from build123d import *

# Parameters (mm, degrees)
SM_BASE_FLANGE_1_DEPTH    = 185
CUT_EXTRUDE_1_REACH       = 197.768
SKETCH_6_R                = 5
SM_EDGE_FLANGE_1_DEPTH    = 49.2634
HOLE_WIZARD_M3_2_D        = 3
CUT_EXTRUDE_START         = -2.7366
CUT_EXTRUDE_6_OUTLINE_W   = 21
CUT_EXTRUDE_6_OUTLINE_H   = 20
CUT_EXTRUDE_6_OUTLINE_H_2 = 19.2634
CUT_EXTRUDE_6_DEPTH       = 2.7366
HOLE_WIZARD_3_5_3_5_1_D   = 3.5
HOLE_WIZARD_7_0_7_1_D     = 7
HOLE_WIZARD_7_0_7_1_DEPTH = 6
HOLE_WIZARD_7_0_7_1_TIP   = 2.103012167
M3X0_5_1_D                = 2.5


# Read off the part's stored shape, not the designer's step: 除料-伸長6
# Sheet-metal steps are written as plain solids
with BuildPart() as part:
    # Sketch 1 → 基材-凸緣1 (new body)
    with BuildSketch(Plane.XY):
        with BuildLine():
            Line((0, -50), (0, -0.7366))
            ThreePointArc((0, -0.7366), (-0.215745145, -0.215745145), (-0.7366, 0))
            Line((-0.7366, 0), (-40, 0))
            Line((-40, 0), (-40, 2))
            Line((-40, 2), (-0.7366, 2))
            ThreePointArc((-0.7366, 2), (1.198468417, 1.198468417), (2, -0.7366))
            Line((2, -0.7366), (2, -50))
            Line((2, -50), (0, -50))
        make_face()
    extrude(amount=SM_BASE_FLANGE_1_DEPTH)

    # 草圖6 → 除料-伸長1 (cut, up to next)
    with BuildSketch(Plane.ZY, mode=Mode.PRIVATE) as cut_extrude_1_sk1:
        with Locations(Location((170, -25, 0), (0, 0, 270))):
            Circle(SKETCH_6_R)
    cut_extrude_1_tool1 = extrude(cut_extrude_1_sk1.sketch, amount=-CUT_EXTRUDE_1_REACH, mode=Mode.PRIVATE) & part.part
    # 草圖6 → 除料-伸長1 (cut, up to next)
    with BuildSketch(Plane.ZY, mode=Mode.PRIVATE) as cut_extrude_1_sk2:
        with BuildLine():
            Line((37, -12), (43, -12))
            ThreePointArc((43, -12), (56, -25), (43, -38))
            Line((43, -38), (37, -38))
            ThreePointArc((37, -38), (24, -25), (37, -12))
        make_face()
    cut_extrude_1_tool2 = extrude(cut_extrude_1_sk2.sketch, amount=-CUT_EXTRUDE_1_REACH, mode=Mode.PRIVATE) & part.part
    # 草圖6 → 除料-伸長1 (cut, up to next)
    with BuildSketch(Plane.ZY, mode=Mode.PRIVATE) as cut_extrude_1_sk3:
        with BuildLine():
            Line((58, -8.25), (64, -8.25))
            ThreePointArc((64, -8.25), (65.75, -10), (64, -11.75))
            Line((64, -11.75), (58, -11.75))
            ThreePointArc((58, -11.75), (56.25, -10), (58, -8.25))
        make_face()
    cut_extrude_1_tool3 = extrude(cut_extrude_1_sk3.sketch, amount=-CUT_EXTRUDE_1_REACH, mode=Mode.PRIVATE) & part.part
    # 草圖6 → 除料-伸長1 (cut, up to next)
    with BuildSketch(Plane.ZY, mode=Mode.PRIVATE) as cut_extrude_1_sk4:
        with BuildLine():
            Line((16, -8.25), (22, -8.25))
            ThreePointArc((22, -8.25), (23.75, -10), (22, -11.75))
            Line((22, -11.75), (16, -11.75))
            ThreePointArc((16, -11.75), (14.25, -10), (16, -8.25))
        make_face()
    cut_extrude_1_tool4 = extrude(cut_extrude_1_sk4.sketch, amount=-CUT_EXTRUDE_1_REACH, mode=Mode.PRIVATE) & part.part
    # 草圖6 → 除料-伸長1 (cut, up to next)
    with BuildSketch(Plane.ZY, mode=Mode.PRIVATE) as cut_extrude_1_sk5:
        with BuildLine():
            Line((16, -38.25), (22, -38.25))
            ThreePointArc((22, -38.25), (23.75, -40), (22, -41.75))
            Line((22, -41.75), (16, -41.75))
            ThreePointArc((16, -41.75), (14.25, -40), (16, -38.25))
        make_face()
    cut_extrude_1_tool5 = extrude(cut_extrude_1_sk5.sketch, amount=-CUT_EXTRUDE_1_REACH, mode=Mode.PRIVATE) & part.part
    # 草圖6 → 除料-伸長1 (cut, up to next)
    with BuildSketch(Plane.ZY, mode=Mode.PRIVATE) as cut_extrude_1_sk6:
        with BuildLine():
            Line((58, -38.25), (64, -38.25))
            ThreePointArc((64, -38.25), (65.75, -40), (64, -41.75))
            Line((64, -41.75), (58, -41.75))
            ThreePointArc((58, -41.75), (56.25, -40), (58, -38.25))
        make_face()
    cut_extrude_1_tool6 = extrude(cut_extrude_1_sk6.sketch, amount=-CUT_EXTRUDE_1_REACH, mode=Mode.PRIVATE) & part.part
    add(cut_extrude_1_tool1.solids().sort_by_distance((0, -25, 170))[0], mode=Mode.SUBTRACT)
    add(cut_extrude_1_tool2.solids().sort_by_distance((0, -25, 40))[0], mode=Mode.SUBTRACT)
    add(cut_extrude_1_tool3.solids().sort_by_distance((0, -10, 61))[0], mode=Mode.SUBTRACT)
    add(cut_extrude_1_tool4.solids().sort_by_distance((0, -10, 19))[0], mode=Mode.SUBTRACT)
    add(cut_extrude_1_tool5.solids().sort_by_distance((0, -40, 19))[0], mode=Mode.SUBTRACT)
    add(cut_extrude_1_tool6.solids().sort_by_distance((0, -40, 61))[0], mode=Mode.SUBTRACT)

    # 邊線-凸緣1 section (across the edge) → 邊線-凸緣1 (add)
    with BuildSketch(Plane(origin=(0, -0.7366, -0.7366), x_dir=(0, 0, 1), z_dir=(0, -1, 0))):
        with BuildLine():
            Line((-2, 0.7366), (-2, 18))
            Line((-2, 18), (0, 18))
            Line((0, 18), (0, 0.7366))
            ThreePointArc((0, 0.7366), (0.215745145, 0.215745145), (0.7366, 0))
            Line((0.7366, 0), (0.7366, -2))
            ThreePointArc((0.7366, -2), (-1.198468417, -1.198468417), (-2, 0.7366))
        make_face()
    extrude(amount=SM_EDGE_FLANGE_1_DEPTH)

    # M3 螺紋孔2 (through all)
    with Locations(Plane(origin=(0, 0, 0), x_dir=(-1, 0, 0), z_dir=(0, -1, 0))):
        with Locations((35, -5), (35, -180), (5, -5), (5, -180)):
            Hole(HOLE_WIZARD_M3_2_D / 2)

    # 除料-伸長6 outline → 除料-伸長6 (cut)
    with BuildSketch(Plane(origin=(0, 0, -2.7366), x_dir=(-1, 0, 0), z_dir=(0, 0, -1)).offset(CUT_EXTRUDE_START)):
        with Locations((7.5, -40)):
            Rectangle(CUT_EXTRUDE_6_OUTLINE_W, CUT_EXTRUDE_6_OUTLINE_H)
        with Locations((7.5, -10.3683)):
            Rectangle(CUT_EXTRUDE_6_OUTLINE_W, CUT_EXTRUDE_6_OUTLINE_H_2)
    extrude(amount=CUT_EXTRUDE_6_DEPTH, mode=Mode.SUBTRACT)

    # Ø3.5 (3.5) 直徑孔1 (through all)
    with Locations(Plane(origin=(0, 0, -2.7366), x_dir=(-1, 0, 0), z_dir=(0, 0, -1))):
        with Locations((15, -25)):
            Hole(HOLE_WIZARD_3_5_3_5_1_D / 2)

    # Ø7.0 (7) 直徑孔1
    with Locations(Plane(origin=(0, 0, 0), x_dir=(-1, 0, 0), z_dir=(0, -1, 0))):
        with Locations((20, -165), (20, -92.5), (20, -12)):
            Hole(HOLE_WIZARD_7_0_7_1_D / 2, depth=HOLE_WIZARD_7_0_7_1_DEPTH)
            with Locations((0, 0, -(HOLE_WIZARD_7_0_7_1_DEPTH + HOLE_WIZARD_7_0_7_1_TIP / 2))):  # 118° drill point
                Cone(0, HOLE_WIZARD_7_0_7_1_D / 2, HOLE_WIZARD_7_0_7_1_TIP, mode=Mode.SUBTRACT)

    # M3x0.5 螺紋孔1 (through all)
    with Locations(Plane(origin=(2, 0, 0), x_dir=(0, 0, -1), z_dir=(1, 0, 0))):
        with Locations((-95, -25), (-87, -25)):
            Hole(M3X0_5_1_D / 2)


solid = part.part
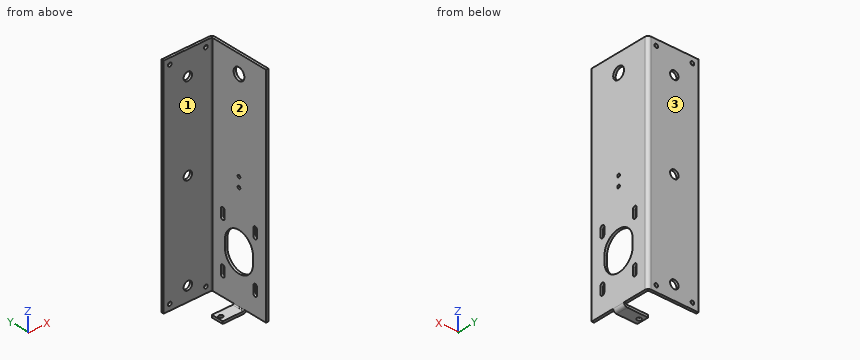
Read the model definition and answer for the solid it produces. Units are mm, in the model's axes. Face numbers are marked on the shaded views. A direction names the side the tool comes from. Coordinates: 2 decimals unless noted, no trailing zeros. Loops run counter-clockwise (first coordinate to the right, second up) from the corner with the lowest first, then second, coordinate; pieces in that order, holes last.
Q1. The part is cut by section B-B on y = -35.5. Write down the section's boundary in (x, z), and give its area (3 significant figures).
Q2. The part is cut by section C-C on z = 81. Write down the section's boundary in (x, y), and give its area (3 significant figures).
Q3. The part is cut by section D-D on x = -30.5. Write down the section's boundary in (y, z).
Q4. Each of these flat-tipped pins is pushed along its axis until it touches: pin 1 Ø4.5 at (x, y) = (-15, -25) entering from +Z; pin 2 Ø8 at (x, z) = (-25, 151.5) entering from -Y; pin 3 Ø0.6 at (y, z) = (-26, -1.5) entering from -X; pin 4 Ø6 at (x, y) = (-30.5, -4) entering from +Z. Where does it stop, or does it pass through?
Q5. Consider probe 1 along X at (y, z) = (1.4, 180); probe 2 along Y at (x, z) = (-19.5, 76.5); probe 3 along Y at (x, z) = (-15, -1.85). Determine where each line is inside the solid, lowest interval first.
Q6. Which of the six approach directions +Z, -Z, +X, -X, +Y, -Y give full straight-line access (tool end or side, diameter ignored) to the marked faces 1, 2 and 3?
Q7. The part is cut by section A-A on x = -10. Write down the section's boundary in (y, z).
Results below:
1. outline: (0, 0) - (2, 0) - (2, 29.34) - (0, 29.34) - close; (0, 50.66) - (2, 50.66) - (2, 185) - (0, 185) - close
1. area: 327 mm2
2. outline: (-40, 0) - (-0.74, 0) arc R0.74 cw to (0, -0.74) - (0, -50) - (2, -50) - (2, -0.74) arc R2.74 ccw to (-0.74, 2) - (-40, 2) - close
2. area: 183 mm2
3. outline: (0, 0) - (2, 0) - (2, 185) - (0, 185) - close
4. pin 1: stops at z = -0.74
4. pin 2: stops at y = 0
4. pin 3: stops at x = -18
4. pin 4: passes through
5. probe 1: x = -40 to -36.5, -33.5 to -6.5, -3.5 to 0.97
5. probe 2: y = 0 to 2
5. probe 3: y = -30 to -26.75, -23.25 to -20
6. face 1: +Z, -Z, -X, -Y
6. face 2: +Z, -X, -Y
6. face 3: +Z, -Z, +X, -X, +Y
7. outline: (-30, -2.74) - (-20, -2.74) - (-20, -0.74) - (-30, -0.74) - close; (0, 0) - (2, 0) - (2, 185) - (0, 185) - close
